from build123d import *

# Parameters (mm, degrees)
SKETCH1_R           = 2.032
BOSS_EXTRUDE1_DEPTH = 13.08
SKETCH2_R           = 2.286
BOSS_EXTRUDE2_DEPTH = 2.54
CUT_EXTRUDE1_DEPTH  = 2.032


with BuildPart() as part:
    # Sketch1 → Boss-Extrude1 (new body)
    with BuildSketch(Plane.XY):
        Circle(SKETCH1_R)
    extrude(amount=BOSS_EXTRUDE1_DEPTH)

    # Sketch2 → Boss-Extrude2 (add)
    with BuildSketch(Plane(origin=(0, 0, 0), x_dir=(-1, 0, 0), z_dir=(0, 0, -1))):
        Circle(SKETCH2_R)
    extrude(amount=BOSS_EXTRUDE2_DEPTH)

    # Sketch3 → Cut-Extrude1 (cut)
    with BuildSketch(Plane(origin=(0, 0, -2.54), x_dir=(-1, 0, 0), z_dir=(0, 0, -1))):
        Polygon((0, -1.554742097), (1.346446152, -0.777371048), (1.346446152, 0.777371048), (0, 1.554742097), (-1.346446152, 0.777371048), (-1.346446152, -0.777371048), align=None)
    extrude(amount=-CUT_EXTRUDE1_DEPTH, mode=Mode.SUBTRACT)


solid = part.part
Check sheet for the modelled part. Datum: model origin and axes. Units: mm. A direction names the side the tool comes from. Round coordinates to 2 decimals unless told otherwise and drop trailing zeros. Loops run counter-clockwise (first coordinate to the right, second up) from the corner with the lowest first, then second, coordinate; pieces in that order, holes last. Notation, with made-up numbers: (49, 19.5) -> (86, 19.5) arc R6 cw to (86, 30.5) -> close; hole circle Ø2 at (-3, 26.25). An arc over 180 degrees is marked (long way). Put each result on its own line as item: value. Start each with the question number.
1. Section check B-B (x = -0.65). Enter the section's corners in (y, z).
2. Section check A-A (y = 0). Enter the section's corners in (x, z), plus the area to 3 significant figures.
3. Access from +Z, -Z, +X, -X, +Y, -Y to the whole of each face (thin tool, end or side, straight path). Record for faces 5 (the face through (0, 0, 13.08)), 6 (the face through (-0.44, -1.984, 6.448)), 7 (the face through (1.346, 0, -2)).
4. Section check C-C (z = 11.75). Enter the section's corners in (x, y).
5. Draft check along X on faces 1 (the face through (0.664, 1.171, -1.538)), 2 (the face through (-1.5, 0, -2.54)), 3 (the face through (0.5, -2.23, -1.25)), 4 (the face through (0, 0, -0.508)). Enter one of: +X half, -X half, draft (parallel to the pull), parting line (faces both ways), or undercut.
6. Section check D-D (y = 1.8). Enter the section's corners in (x, z), plus the area to 3 significant figures.
7. Scan lines: probe 1 along Z at (x, y) = (0.95, 0.75); probe 2 along Z at (x, y) = (1.2, -1.7); probe 3 along Y at (x, z) = (-0.85, 4). Record each from-to range of solid material in increasing order.
Findings:
1. outline: (-2.19, -2.54) -> (-1.18, -2.54) -> (-1.18, -0.51) -> (1.18, -0.51) -> (1.18, -2.54) -> (2.19, -2.54) -> (2.19, 0) -> (1.93, 0) -> (1.93, 13.08) -> (-1.93, 13.08) -> (-1.93, 0) -> (-2.19, 0) -> close
2. outline: (-2.29, -2.54) -> (-1.35, -2.54) -> (-1.35, -0.51) -> (1.35, -0.51) -> (1.35, -2.54) -> (2.29, -2.54) -> (2.29, 0) -> (2.03, 0) -> (2.03, 13.08) -> (-2.03, 13.08) -> (-2.03, 0) -> (-2.29, 0) -> close
2. area: 59.3 mm^2
3. face 5: +Z, +X, -X, +Y, -Y
3. face 6: +Z
3. face 7: -Z
4. outline: circle Ø4.06 at (0, 0)
5. face 1: undercut
5. face 2: draft
5. face 3: parting line
5. face 4: undercut
6. outline: (-1.41, -2.54) -> (1.41, -2.54) -> (1.41, 0) -> (0.94, 0) -> (0.94, 13.08) -> (-0.94, 13.08) -> (-0.94, 0) -> (-1.41, 0) -> close
6. area: 31.8 mm^2
7. probe 1: z = -0.51 to 13.08
7. probe 2: z = -2.54 to 0
7. probe 3: y = -1.85 to 1.85
